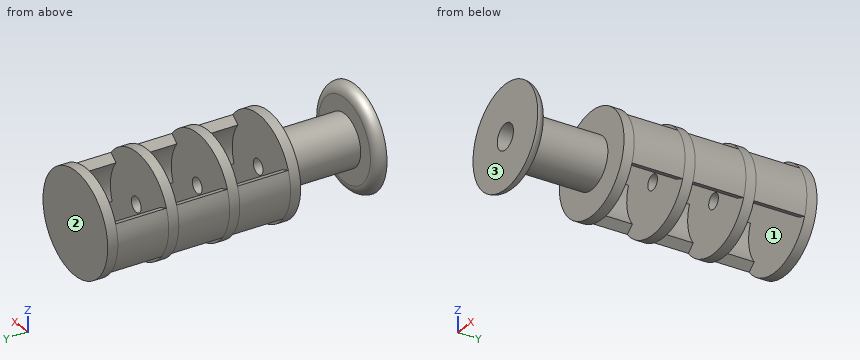
```python
from build123d import *

# Parameters (mm, degrees)
CROQUIS1_R               = 5
SALIENTE_EXTRUIR1_DEPTH  = 15
CROQUIS1_3_R             = 10
CROQUIS1_3_R_2           = 5
SALIENTE_EXTRUIR2_DEPTH  = 2
CROQUIS2_R               = 10
SALIENTE_EXTRUIR3_DEPTH  = 2
SALIENTE_EXTRUIR4_DEPTH  = 10
CROQUIS4_R               = 10
SALIENTE_EXTRUIR5_DEPTH  = 2
SALIENTE_EXTRUIR6_START  = 12
SALIENTE_EXTRUIR6_DEPTH  = 10
CROQUIS5_R               = 10
SALIENTE_EXTRUIR7_DEPTH  = 2
SALIENTE_EXTRUIR8_START  = 24
SALIENTE_EXTRUIR8_DEPTH  = 10
CROQUIS7_R               = 10
SALIENTE_EXTRUIR9_DEPTH  = 2
CORTAR_EXTRUIR1_REACH    = 56.854
CROQUIS9_R               = 1.5
SALIENTE_EXTRUIR10_START = 2
CROQUIS10_R              = 5
CROQUIS10_R_2            = 1.5
SALIENTE_EXTRUIR10_DEPTH = 2
CROQUIS11_R              = 2.5
CORTAR_EXTRUIR2_DEPTH    = 15
REDONDEO1_R              = 2


with BuildPart() as part:
    # Croquis1 → Saliente-Extruir1 (new body)
    with BuildSketch(Plane(origin=(0, 0, 0), x_dir=(1, 0, 0), z_dir=(0, 1, 0))):
        with Locations(Location((0, 0, 0), (0, 0, 270))):
            Circle(CROQUIS1_R)
    extrude(amount=SALIENTE_EXTRUIR1_DEPTH)

    # Croquis2 → Saliente-Extruir3 (add)
    with BuildSketch(Plane(origin=(0, 15, 0), x_dir=(1, 0, 0), z_dir=(0, 1, 0))):
        with Locations(Location((0, 0, 0), (0, 0, 270))):
            Circle(CROQUIS2_R)
    extrude(amount=SALIENTE_EXTRUIR3_DEPTH)

    # Croquis3 → Saliente-Extruir4 (add)
    with BuildSketch(Plane(origin=(0, 17, 0), x_dir=(1, 0, 0), z_dir=(0, 1, 0))):
        with BuildLine():
            Line((-6.254092926, 4.988619216), (-7.817616157, 6.235774019))
            ThreePointArc((-7.817616157, 6.235774019), (-9.888141199, 1.491530635), (-9.309146792, -3.652367179))
            Line((-9.309146792, -3.652367179), (-7.447317433, -2.921893743))
            ThreePointArc((-7.447317433, -2.921893743), (-7.910512959, 1.193224508), (-6.254092926, 4.988619216))
        make_face()
        with BuildLine():
            ThreePointArc((7.817616157, -6.235774019), (9.888141199, -1.491530635), (9.309146792, 3.652367179))
            Line((9.309146792, 3.652367179), (7.447317433, 2.921893743))
            ThreePointArc((7.447317433, 2.921893743), (7.910512959, -1.193224508), (6.254092926, -4.988619216))
            Line((6.254092926, -4.988619216), (7.817616157, -6.235774019))
        make_face()
    extrude(amount=SALIENTE_EXTRUIR4_DEPTH)

    # Croquis4 → Saliente-Extruir5 (add)
    with BuildSketch(Plane(origin=(0, 27, 0), x_dir=(1, 0, 0), z_dir=(0, 1, 0))):
        with Locations(Location((0, 0, 0), (0, 0, 270))):
            Circle(CROQUIS4_R)
    extrude(amount=SALIENTE_EXTRUIR5_DEPTH)

    # Croquis3<3> → Saliente-Extruir6 (add)
    with BuildSketch(Plane(origin=(0, 17, 0), x_dir=(1, 0, 0), z_dir=(0, 1, 0)).offset(SALIENTE_EXTRUIR6_START)):
        with BuildLine():
            Line((-6.254092926, 4.988619216), (-7.817616157, 6.235774019))
            ThreePointArc((-7.817616157, 6.235774019), (-9.888141199, 1.491530635), (-9.309146792, -3.652367179))
            Line((-9.309146792, -3.652367179), (-7.447317433, -2.921893743))
            ThreePointArc((-7.447317433, -2.921893743), (-7.910512959, 1.193224508), (-6.254092926, 4.988619216))
        make_face()
        with BuildLine():
            ThreePointArc((7.817616157, -6.235774019), (9.888141199, -1.491530635), (9.309146792, 3.652367179))
            Line((9.309146792, 3.652367179), (7.447317433, 2.921893743))
            ThreePointArc((7.447317433, 2.921893743), (7.910512959, -1.193224508), (6.254092926, -4.988619216))
            Line((6.254092926, -4.988619216), (7.817616157, -6.235774019))
        make_face()
    extrude(amount=SALIENTE_EXTRUIR6_DEPTH)

    # Croquis5 → Saliente-Extruir7 (add)
    with BuildSketch(Plane(origin=(0, 39, 0), x_dir=(1, 0, 0), z_dir=(0, 1, 0))):
        with Locations(Location((0, 0, 0), (0, 0, 270))):
            Circle(CROQUIS5_R)
    extrude(amount=SALIENTE_EXTRUIR7_DEPTH)

    # Croquis3<4> → Saliente-Extruir8 (add)
    with BuildSketch(Plane(origin=(0, 17, 0), x_dir=(1, 0, 0), z_dir=(0, 1, 0)).offset(SALIENTE_EXTRUIR8_START)):
        with BuildLine():
            Line((-6.254092926, 4.988619216), (-7.817616157, 6.235774019))
            ThreePointArc((-7.817616157, 6.235774019), (-9.888141199, 1.491530635), (-9.309146792, -3.652367179))
            Line((-9.309146792, -3.652367179), (-7.447317433, -2.921893743))
            ThreePointArc((-7.447317433, -2.921893743), (-7.910512959, 1.193224508), (-6.254092926, 4.988619216))
        make_face()
        with BuildLine():
            ThreePointArc((7.817616157, -6.235774019), (9.888141199, -1.491530635), (9.309146792, 3.652367179))
            Line((9.309146792, 3.652367179), (7.447317433, 2.921893743))
            ThreePointArc((7.447317433, 2.921893743), (7.910512959, -1.193224508), (6.254092926, -4.988619216))
            Line((6.254092926, -4.988619216), (7.817616157, -6.235774019))
        make_face()
    extrude(amount=SALIENTE_EXTRUIR8_DEPTH)

    # Croquis7 → Saliente-Extruir9 (add)
    with BuildSketch(Plane(origin=(0, 51, 0), x_dir=(1, 0, 0), z_dir=(0, 1, 0))):
        with Locations(Location((0, 0, 0), (0, 0, 270))):
            Circle(CROQUIS7_R)
    extrude(amount=SALIENTE_EXTRUIR9_DEPTH)

    # Cortar-Extruir1: up to this face of the body (flat: up to its plane)
    cortar_extruir1_end = Plane(part.part.faces().sort_by_distance((0, 51, 0))[0])
    # Croquis9 → Cortar-Extruir1 (cut, up to the picked face)
    with BuildSketch(Plane.XZ, mode=Mode.PRIVATE) as cortar_extruir1_sk1:
        with Locations(Location((0, 0, 0), (0, 0, 90))):
            Circle(CROQUIS9_R)
    cortar_extruir1_tool1 = split(extrude(cortar_extruir1_sk1.sketch, amount=-CORTAR_EXTRUIR1_REACH, mode=Mode.PRIVATE), bisect_by=cortar_extruir1_end, keep=Keep.BOTH, mode=Mode.PRIVATE)
    add(cortar_extruir1_tool1.solids().sort_by(Axis((0, 0, 0), (0, 1, 0)))[0], mode=Mode.SUBTRACT)



with BuildPart() as body_2:
    # Croquis1<3> → Saliente-Extruir2 (new body)
    with BuildSketch(Plane(origin=(0, 0, 0), x_dir=(1, 0, 0), z_dir=(0, 1, 0))):
        with Locations(Location((0, 0, 0), (0, 0, 270))):
            Circle(CROQUIS1_3_R)
        with Locations(Location((0, 0, 0), (0, 0, 270))):
            Circle(CROQUIS1_3_R_2, mode=Mode.SUBTRACT)
    extrude(amount=-SALIENTE_EXTRUIR2_DEPTH)


with BuildPart() as part_1:
    add(part.part)

    add(body_2.part)  # Saliente-Extruir10 merges body 2
    # Croquis10 → Saliente-Extruir10 (add)
    with BuildSketch(Plane.XZ.offset(SALIENTE_EXTRUIR10_START)):
        with Locations(Location((0, 0, 0), (0, 0, 90))):
            Circle(CROQUIS10_R)
        with Locations(Location((0, 0, 0), (0, 0, 90))):
            Circle(CROQUIS10_R_2, mode=Mode.SUBTRACT)
    extrude(amount=-SALIENTE_EXTRUIR10_DEPTH)

    # Croquis11 → Cortar-Extruir2 (cut)
    with BuildSketch(Plane.XZ.offset(2)):
        with Locations(Location((0, 0, 0), (0, 0, 270))):
            Circle(CROQUIS11_R)
    extrude(amount=-CORTAR_EXTRUIR2_DEPTH, mode=Mode.SUBTRACT)

    # Redondeo1
    redondeo1_edges = [part_1.edges().sort_by_distance(p)[0] for p in [
        (0, 0, -10),
    ]]
    fillet(redondeo1_edges, radius=REDONDEO1_R - 0.0001)  # a hair under: the kernel refuses the full size


solid = part_1.part
```
The model under review builds one solid part; all positions refer to its coordinate system, in mm. Face numbers are marked on the shaded views. Give positions to 0.01 mm unless a question says otherwise; leave off trailing zeros. Write each loop counter-clockwise with the first axis right and the second up, starting at its lowest first coordinate (ties: lowest second). Pieces come first, ordered by that corner, then holes. Notation, with made-up numbers: M 49,-4 L 57,-4 A20 cw 57,7 Z; hole C -24,29 d3. An arc over 180 degrees is marked long. Write item = value, one per line. Start each with the question number.
Q1. We need section C-C (y = 2). State the section outline as (x, z) points, plus the area to 3 significant figures.
Q2. Mouldability with a two-part tool opening along Y and no side actions: class the marked faces 1, 2 and 3 as released by +Y, released by -Y, zero draft, split by the parting line, or undercut.
Q3. Clearance check with flat-ended pins moving along their axes: pin 1 (3 mm diameter, centred on x = -4.5, y = 13, fed in from +Z); pin 2 (2.5 mm diameter, centred on x = 0.5, z = 0.5, fed in from -Y); pin 3 (5 mm diameter, centred on x = 5.5, y = 39, fed in from -Z). State where each tip first meets the part, or that it passes through.
Q4. We need section B-B (x = 0). Give the number of separate pieces and of enclosed holes in the cut face, plus the area to 3 significant figures.
Q5. We need section A-A (y = 24.5). State the section outline as (x, z) points.
Q6. For line 1 (Y direction, x = 2, z = -5.5); line 2 (Y direction, x = 1.5, z = 1); line 3 (Y direction, x = -2, z = 4.25), list the stretches that pass through material, from the lowest coordinate up.
Result set:
q1.outline = C 0,0 d10; hole C 0,0 d5
q1.area = 58.9 mm2
q2.face_1 = undercut
q2.face_2 = released by +Y
q2.face_3 = released by -Y
q3.pin_1 = 4
q3.pin_2 = 13
q3.pin_3 = -9.54
q4.separate_pieces = 7
q4.enclosed_holes = 0
q4.area = 249 mm2
q5.outline = M -9.31,3.65 A10 ccw -7.82,-6.24 L -6.25,-4.99 A8 cw -7.45,2.92 Z; M 6.25,4.99 A8 cw 7.45,-2.92 L 9.31,-3.65 A10 ccw 7.82,6.24 Z
q6.line_1 = -2 to 0, 15 to 17, 27 to 29, 39 to 41, 51 to 53
q6.line_2 = 13 to 17, 27 to 29, 39 to 41, 51 to 53
q6.line_3 = -2 to 17, 27 to 29, 39 to 41, 51 to 53
